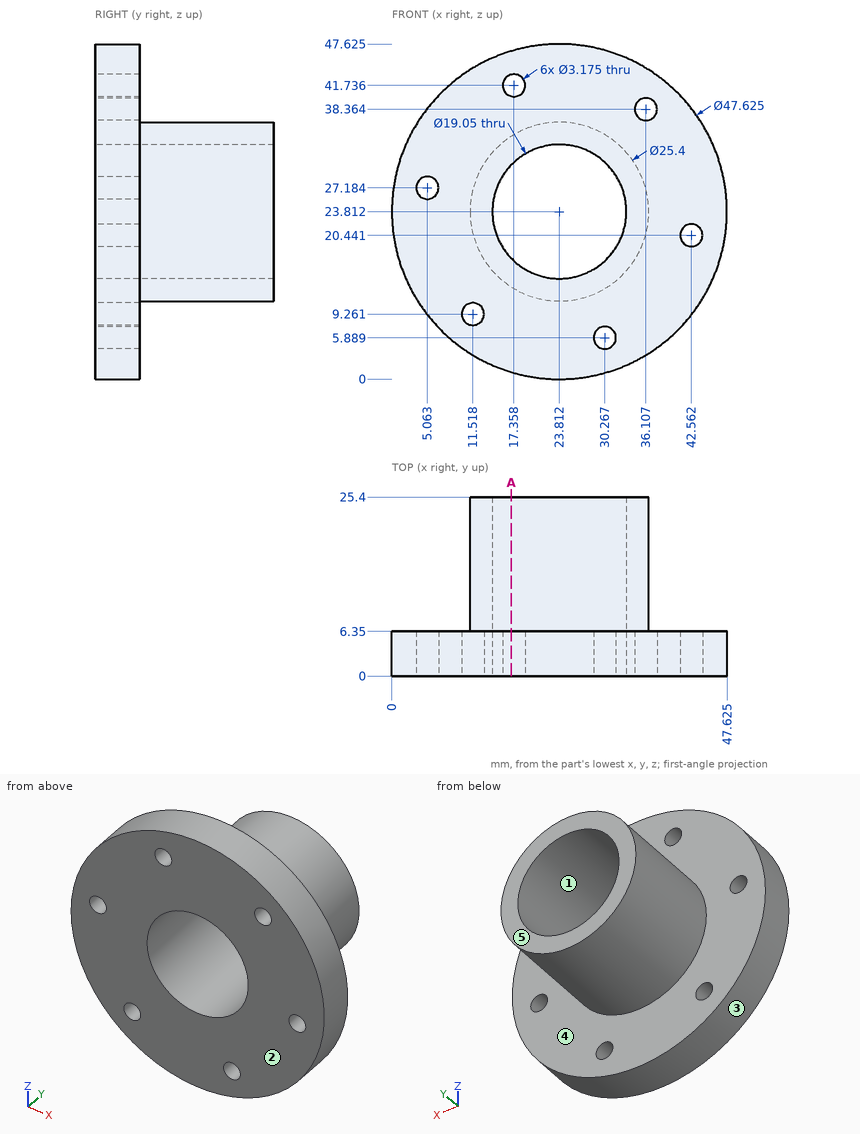
Design review of the part shown in the three views and the two pictorial views. Dimensions are in mm from the part's minimum x, y and z. A direction names the side the tool comes from. Give positions to 0.01 mm unless a question says otherwise; leave off trailing zeros. Write item = value, one per line.
1) Take a section at A-A on x = 17. Count the separate pieces of the cut face and the enclosed holes in it, and give its area (3 significant figures).
Result sheet:
separate_pieces = 3
enclosed_holes = 0
area = 340 mm2
2) Tool access review of the marked faces 4 and 5: name each direction out of +Z, -Z, +X, -X, +Y, -Y from which nothing blocks a thin tool from reaching the whole face with its end or side.
Result sheet:
face_4 = +Y
face_5 = +Z, -Z, +X, -X, +Y
3) Draft analysis for pull direction Z (two halves, no side actions). For the marked faces 1, 2 and 3, state which applies: +Z half, -Z half, draft (parallel to the pull), parting line (faces both ways), or undercut.
Result sheet:
face_1 = undercut
face_2 = draft
face_3 = parting line
4) Clearance check with flat-ended pins moving along their axes: pin 1 Ø5 at (y, z) = (6, 31) entering from -X; pin 2 Ø4 at (x, z) = (17.36, 41.74) entering from +Y; pin 3 Ø8 at (x, y) = (36.5, 22.5) entering from +Z (1 decimal). State where each tip first meets the part, or that it passes through.
Result sheet:
pin_1 = 0.47
pin_2 = 6.35
pin_3 = 33.1
5) To check wall thickness, follow line 1 (X direction, y = 5.5, z = 27) (1 decimal); line 2 (Y direction, x = 7, z = 34); line 3 (Z direction, x = 23.5, y = 10.75). State the ranges of each line that lie inside material, in increasing order.
Result sheet:
line_1 = 0.2 to 3.5, 6.6 to 14.8, 32.8 to 47.4
line_2 = 0 to 6.35
line_3 = 11.12 to 14.29, 33.33 to 36.51
